Autodesk Inventor part; units mm, degrees
ref_plane "YZ Plane" through (0, 0, 0) normal (1, 0, 0) x (0, 1, 0)
ref_plane "XZ Plane" through (0, 0, 0) normal (0, 1, 0) x (-1, 0, 0)
ref_plane "XY Plane" through (0, 0, 0) normal (0, 0, 1) x (1, 0, 0)
sketch "Sketch1" plane through (0, 0, 0) normal (0, 0, 1) x (1, 0, 0)
  arc A0 (-6.3312, 9.4953) -> (-1.2535, 11.3435) centre (0, 0) ccw
  arc A1 (-39.762, 56.0914) -> (-36.7433, 54.5415) centre (-40.9824, 50) ccw
  arc A2 (-35.5994, 53.3683) -> (-45.7281, 45.7808) centre (-40.9824, 50) ccw
  arc A3 (-9.826, -6.7195) -> (7.1791, 9.4953) centre (0, 0) ccw
  line L0 (-45.7281, 45.7808) -> (-9.826, -6.7195)
  line L1 (-36.7433, 54.5415) -> (-36.3354, 54.1231)
  line L2 (-35.5994, 53.3683) -> (7.1791, 9.4953)
  arc A4 (-10.3384, -7.0699) -> (7.5913, 9.9618) centre (0, 0) ccw
  line L3 (-10.3384, -7.0699) -> (-46.2188, 45.3986)
  arc A5 (-35.1095, 53.7552) -> (-46.2188, 45.3986) centre (-40.9824, 50) ccw
  line L4 (-35.1095, 53.7552) -> (7.5913, 9.9618)
  point P0 (0, 0)
  dimension "d0" = 12.7
extrude "Extrusion1" add sketch "Sketch1" along normal blind 6.35 contours L3 A5 L4 A4
properties part number "z-belt"
Can you work these out from the model? Positions are in its coordinate system, mm. A direction names the side the tool comes from. Coordinates: 2 decimals unless noted, no trailing zeros. Order: outer loops, then holes, each group sorted by start corner. A loop starts at its lowest first (then second) coordinate and runs counter-clockwise, first axis right, second up.
1. I need wall thicknesses on line 1 (X direction, y = 26, z = 1); line 2 (Y direction, x = -2.5, z = 3.25); line 3 (X direction, y = -8, z = 4). Which ranges of each line are inside material? Lowest first, please.
2. Thinking about a two-plate mould opening in Y: for faces 3 (the face through (-45.3, 55.473, 3.131)), 4 (the face through (8.421, -8.413, 3.131)), 5 (the face through (-25, 15, 0)), 6 (the face through (-28.03, 18.8, 3.13)), which applies, +Y half, -Y half, draft (parallel to the pull), parting line (faces both ways), or undercut?
3. If we section it at B-B (z = 4): Please give me the cut outline in (x, y).
4. For faces 1 (the face through (-14.058, 32.165, 3.131)), 2 (the face through (-28.03, 19.9, 3.13)), which set-ups out of +Z, -Z, +X, -X, +Y, -Y let a thin tool reach every point of the face, with its end or its side?
5. If we section it at C-C (x = -12): Please give me the cut outline in (y, z), then the cut area to 3 significant figures.
6. I'm going to push flat-ended pins straight in: pin 1 (2 mm diameter, centred on x = -33.5, y = 32, fed in from +Z); pin 2 (3 mm diameter, centred on x = 2, z = 1.5, fed in from +Y); pin 3 (3 mm diameter, centred on x = -37.5, z = 0.5, fed in from -Y). Where does each tip first touch, or does it pass through?
7. If we section it at A-A (y = -4): Please give me the cut outline in (x, z), then the cut area to 3 significant figures.
Entries:
1. line 1: x = -32.95 to -32.2, -8.91 to -8.05
1. line 2: y = -12.27 to -11.64, 19.42 to 20.31
1. line 3: x = -9.64 to -8.81, 8.81 to 9.64
2. face 3: parting line
2. face 4: undercut
2. face 5: draft
2. face 6: -Y half
3. outline: (-46.22, 45.4) - (-10.34, -7.07) arc R12.52 ccw (long way) to (7.59, 9.96) - (-35.11, 53.76) arc R6.97 ccw (long way) to start; hole (-45.73, 45.78) - (-9.83, -6.72) arc R11.9 ccw (long way) to (7.18, 9.5) - (-35.6, 53.37) arc R6.35 ccw (long way) to start
4. face 1: +Z, -Z, +X, +Y
4. face 2: +Z, -Z
5. outline: (-4.64, 0) - (-3.54, 0) - (-3.54, 6.35) - (-4.64, 6.35) - close; (29.17, 0) - (30.05, 0) - (30.05, 6.35) - (29.17, 6.35) - close
5. area: 12.6 mm2
6. pin 1: passes through
6. pin 2: stops at y = 17.23
6. pin 3: stops at y = 30.46
7. outline: (-12.44, 0) - (-11.69, 0) - (-11.69, 6.35) - (-12.44, 6.35) - close; (11.21, 0) - (11.87, 0) - (11.87, 6.35) - (11.21, 6.35) - close
7. area: 8.95 mm2
